Design review of the part shown in the three views and the two pictorial views. Dimensions are in mm from the part's minimum x, y and z. Round coordinates to 2 decimals unless told otherwise and drop trailing zeros. Loops run counter-clockwise (first coordinate to the right, second up) from the corner with the lowest first, then second, coordinate; pieces in that order, holes last.
1. Consider section C-C on z = 2.25. State the section outline as (x, y) points, then the cut area to 3 significant figures.
2. Draft analysis for pull direction X (two halves, no side actions). For the marked faces 1 and 2, state which applies: released by +X, released by -X, zero draft, split by the parting line, or undercut.
3. Consider section B-B on y = 50.5. State the section outline as (x, z) points.
4. Consider section D-D on x = 21. State the section outline as (y, z) points.
5. Consider section A-A on x = 85.5. State the section outline as (y, z) points, then the cut area to 3 significant figures.
6. To check wall thickness, follow line 1 along Z through (x, y) = (68.5, 31.5); line 2 along X through (y, z) = (5, 3.75). State the ranges of each line that lie inside material, in increasing order.
7. Clearance check with flat-ended pins moving along their axes: pin 1 Ø2.5 at (x, z) = (80.5, 5.5) entering from -Y; pin 2 Ø1.5 at (x, z) = (8, 5) entering from +Y; pin 3 Ø2 at (y, z) = (12.5, 3.5) entering from -X; pin 4 Ø2 at (y, z) = (25.5, 4.5) entering from +X. State where each tip first meets the part, or that it passes through.
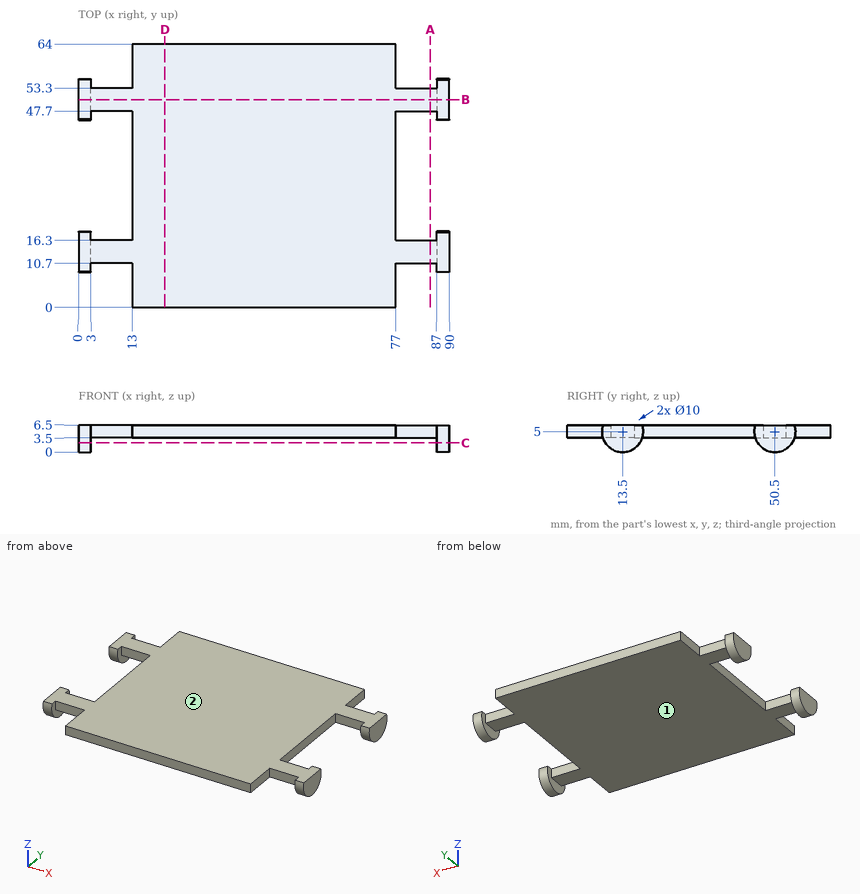
Resolved:
1. outline: (0, 9.32) - (3, 9.32) - (3, 17.68) - (0, 17.68) - close; (0, 46.32) - (3, 46.32) - (3, 54.68) - (0, 54.68) - close; (87, 9.32) - (90, 9.32) - (90, 17.68) - (87, 17.68) - close; (87, 46.32) - (90, 46.32) - (90, 54.68) - (87, 54.68) - close
1. area: 100 mm2
2. face 1: undercut
2. face 2: zero draft
3. outline: (0, 0) - (3, 0) - (3, 3.5) - (87, 3.5) - (87, 0) - (90, 0) - (90, 6.5) - (0, 6.5) - close
4. outline: (0, 3.5) - (64, 3.5) - (64, 6.5) - (0, 6.5) - close
5. outline: (10.7, 3.5) - (16.3, 3.5) - (16.3, 6.5) - (10.7, 6.5) - close; (47.7, 3.5) - (53.3, 3.5) - (53.3, 6.5) - (47.7, 6.5) - close
5. area: 33.6 mm2
6. line 1: z = 3.5 to 6.5
6. line 2: x = 13 to 77
7. pin 1: stops at y = 10.7
7. pin 2: stops at y = 53.3
7. pin 3: stops at x = 0
7. pin 4: stops at x = 77
